```python
from build123d import *

# Parameters (mm, degrees)
SKETCH2_R           = 3
SKETCH4_R           = 3
BOSS_EXTRUDE1_DEPTH = 30
SKETCH5_R           = 3
BOSS_EXTRUDE2_DEPTH = 20


with BuildPart() as part:
    # Sweep1: sweep along a path in Sketch1
    with BuildLine(Plane.XY) as sweep1_path:
        Line((0, 0), (0, 100))
        ThreePointArc((0, 100), (-2.928932188, 107.071067812), (-10, 110))
        Line((-10, 110), (-40.137832809, 110))
        ThreePointArc((-40.137832809, 110), (-44.510528091, 108.993305064), (-48.002829333, 106.175907194))
        Line((-48.002829333, 106.175907194), (-57.405523913, 94.201608056))
    # Sketch2 → Sweep1 (sweep)
    with BuildSketch(Plane(origin=(0, 0, 0), x_dir=(1, 0, 0), z_dir=(0, 1, 0))):
        Circle(SKETCH2_R)
    sweep(path=sweep1_path.line)

    # Sketch4 → Boss-Extrude1 (add)
    with BuildSketch(Plane.XZ):
        Circle(SKETCH4_R)
    extrude(amount=BOSS_EXTRUDE1_DEPTH)

    # Sketch5 → Boss-Extrude2 (add)
    with BuildSketch(Plane.XZ.offset(30)):
        Circle(SKETCH5_R)
    extrude(amount=BOSS_EXTRUDE2_DEPTH)


solid = part.part
```
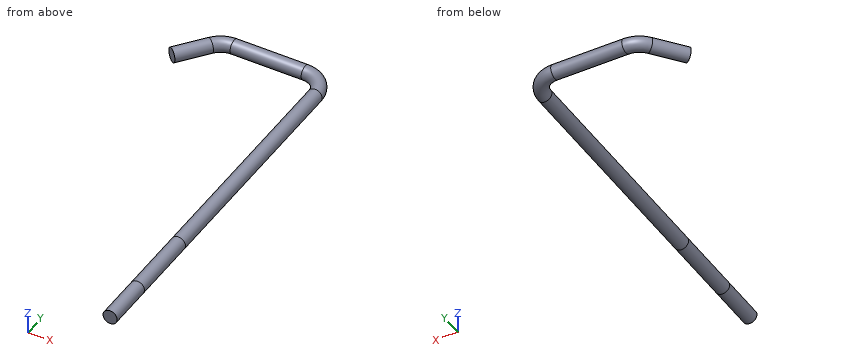
CAD build for the part. Positions are in the model's coordinates, mm. Give positions to 0.01 mm unless a question says otherwise; leave off trailing zeros. Loops run counter-clockwise (first coordinate to the right, second up) from the corner with the lowest first, then second, coordinate; pieces in that order, holes last. Notation, with made-up numbers: (54, 69) - (63, 69) arc R19 cw to (63, 101) - close; hole circle Ø2 at (29.5, 28.25). An arc over 180 degrees is marked (long way). Put each result on its own line as item: value.
Q1. Slice it at B-B (y = 18.5). Give the cut face in (x, z), plus the area to 3 significant figures.
Filled in:
outline: circle Ø6 at (0, 0)
area: 28.3 mm²
Q2. Probe line 1 along X through (y, z) = (98, -1.25); line 2 along X through (y, z) = (28, 0.25); line 3 along X through (y, z) = (32, 2). List the from-to ranges inside material, lowest first.
Filled in:
line 1: x = -57.89 to -50.96, -2.73 to 2.73
line 2: x = -2.99 to 2.99
line 3: x = -2.24 to 2.24
Q3. Flat gauge pins, fed straight in: pin 1 (3 mm diameter, centred on y = 43.5, z = -1.5, fed in from -X); pin 2 (3 mm diameter, centred on x = -27, z = -1, fed in from -Y); pin 3 (2 mm diameter, centred on y = -23.5, z = 1.5, fed in from +X). Where does each tip first touch, or does it go through?
Filled in:
pin 1: stops at x = -3
pin 2: stops at y = 107
pin 3: stops at x = 2.96
Q4. Slice it at A-A (z = -1). Give the cut face in (x, y).
Filled in:
outline: (-59.63, 95.95) - (-55.18, 92.45) - (-45.78, 104.43) arc R7.17 cw to (-40.14, 107.17) - (-10, 107.17) arc R7.17 cw to (-2.83, 100) - (-2.83, -50) - (2.83, -50) - (2.83, 100) arc R12.83 ccw to (-10, 112.83) - (-40.14, 112.83) arc R12.83 ccw to (-50.23, 107.92) - close
